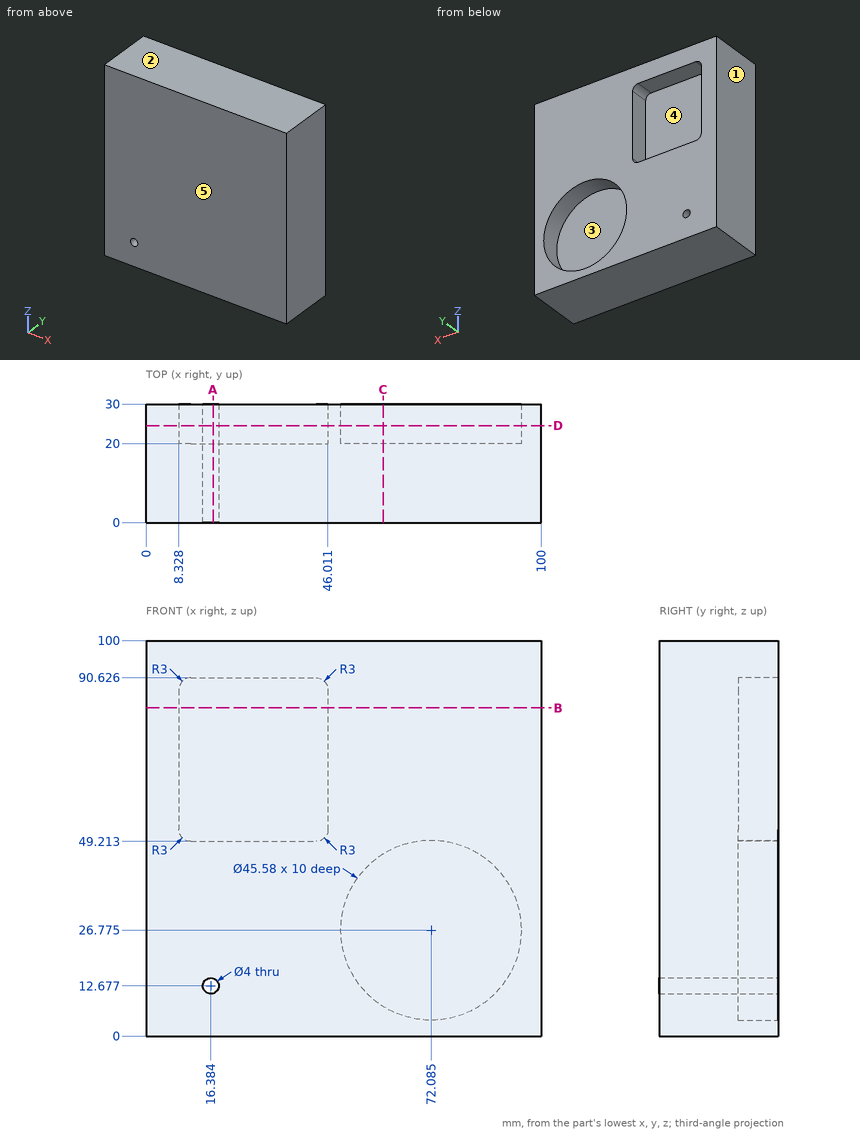
Geometry check sheet. Reference: drawing and pictorial views, mm from the part's lowest x, y, z. A direction names the side the tool comes from. Give positions to 0.01 mm unless a question says otherwise; leave off trailing zeros. Order: outer loops, then holes, each group sorted by start corner. A loop starts at its lowest first (then second) coordinate and runs counter-clockwise, first axis right, second up.
1. Access from +Z, -Z, +X, -X, +Y, -Y to the whole of each face (thin tool, end or side, straight path). Record for the marked faces 4 and 5.
2. Thickness scan on L1, parallel to Z at x = 17.5, y = 28 (1 decimal); L2, parallel to X at y = 23.75, z = 16.5; L3, parallel to X at y = 22.5, z = 82. Record the ranges inside material, lowest first.
3. Section check A-A, the plane x = 17. Enter the section's corners in (y, z), and give its area (3 significant figures).
4. Section check C-C, the plane x = 60. Enter the section's corners in (y, z).
5. Section check B-B, the plane z = 83. Enter the section's corners in (x, y), and give its area (3 significant figures).
6. Release check for a two-part mould opening along Z. For the marked faces 1, 2 and 3 record: pulls with the +Z half, pulls with the -Z half, needs draft (parallel to the pull), parting line crosses it, or undercut.
7. Gauge pin test, flat end, axial feed: pin 1 Ø23 at (x, z) = (73, 37) entering from +Y. Record the tip position at first contact, or that the pin passes through.
8. Section check D-D, the plane y = 24.5. Enter the section's corners in (x, z) (1 decimal).
Values follow:
1. face 4: +Y
1. face 5: +Z, -Z, +X, -X, -Y
2. L1: z = 0 to 11, 14.3 to 49.2, 90.6 to 100
2. L2: x = 0 to 51.74, 92.43 to 100
2. L3: x = 0 to 8.33, 46.01 to 100
3. outline: (0, 0) - (30, 0) - (30, 10.77) - (0, 10.77) - close; (0, 14.58) - (30, 14.58) - (30, 49.21) - (20, 49.21) - (20, 90.63) - (30, 90.63) - (30, 100) - (0, 100) - close
3. area: 2,470 mm2
4. outline: (0, 0) - (30, 0) - (30, 7.45) - (20, 7.45) - (20, 46.1) - (30, 46.1) - (30, 100) - (0, 100) - close
5. outline: (0, 0) - (100, 0) - (100, 30) - (46.01, 30) - (46.01, 20) - (8.33, 20) - (8.33, 30) - (0, 30) - close
5. area: 2,620 mm2
6. face 1: needs draft
6. face 2: pulls with the +Z half
6. face 3: undercut
7. pin 1: stops at y = 20
8. outline: (0, 0) - (100, 0) - (100, 100) - (0, 100) - close; hole (8.3, 52.2) arc R3 ccw to (11.3, 49.2) - (43, 49.2) arc R3 ccw to (46, 52.2) - (46, 87.6) arc R3 ccw to (43, 90.6) - (11.3, 90.6) arc R3 ccw to (8.3, 87.6) - close; hole circle Ø4 at (16.4, 12.7); hole circle Ø45.6 at (72.1, 26.8)
